from build123d import *

# Parameters (mm, degrees)
F1_DEPTH    = 25
F2_SIZE2    = 5
F2_SIZE     = 20
F3_SIZE2    = 5
F3_SIZE     = 20
F4_SIZE2    = 3
F4_SIZE     = 20
F5_SIZE2    = 10
F5_SIZE     = 20
F6_T1_DEPTH = 105.7467241961
F7_R        = 1.5
F13_DEPTH   = 80
F8_R        = 1.5
F14_DEPTH   = 30
F9_R        = 1.5
F15_DEPTH   = 40
F10_R       = 1.5
F16_DEPTH   = 30
F11_R       = 1.5
F17_DEPTH   = 80
F12_R       = 1.5
F18_DEPTH   = 55
F19_R       = 6
F25_DEPTH   = 12
F20_R       = 6
F26_DEPTH   = 12
F21_R       = 6
F27_DEPTH   = 12
F22_R       = 6
F28_DEPTH   = 12
F23_R       = 6
F29_DEPTH   = 12
F24_R       = 6
F30_DEPTH   = 12
F31_R       = 6
F34_D       = 4
F34_DEPTH   = 4
F34_TIP     = 1.2017212381


# Not quite as in the source:
# - a fillet or chamfer that OpenCascade refuses, or shapes differently, is made with other operations: its cross-section is extruded or revolved along the edge and cut away or added


with BuildPart() as f1:
    # F0 (on Top) → F1 (new body)
    with BuildSketch(Plane.XY):
        Polygon((15, 0), (4.6352549156, 14.2658477444), (-12.1352549156, 8.8167787844), (-12.1352549156, -8.8167787844), (4.6352549156, -14.2658477444), align=None)
    extrude(amount=F1_DEPTH)

    # F2
    f2_edges = [f1.edges().sort_by_distance(p)[0] for p in [
        (-3.75, -11.541313, 25),
    ]]
    f2_side = f1.faces().sort_by_distance((-3.75, -11.541313, 12.5))[0]
    chamfer(f2_edges, length=F2_SIZE, length2=F2_SIZE2, reference=f2_side)

    # F3
    f3_edges = [f1.edges().sort_by_distance(p)[0] for p in [
        (11.362712, -5.006297, 25),
    ]]
    f3_side = f1.faces().sort_by_distance((10.379872, -6.359061, 11.710138))[0]
    chamfer(f3_edges, length=F3_SIZE, length2=F3_SIZE2, reference=f3_side)

    # F4
    f4_edges = [f1.edges().sort_by_distance(p)[0] for p in [
        (8.272542, 9.259551, 25),
    ]]
    f4_side = f1.faces().sort_by_distance((9.255383, 7.906786, 11.710138))[0]
    chamfer(f4_edges, length=F4_SIZE, length2=F4_SIZE2, reference=f4_side)

    # F5
    f5_edges = [f1.edges().sort_by_distance(p)[0] for p in [
        (-5.25, 11.053934, 25),
    ]]
    f5_side = f1.faces().sort_by_distance((-4.319172, 11.356378, 12.050432))[0]
    chamfer(f5_edges, length=F5_SIZE, length2=F5_SIZE2, reference=f5_side)

    # F6: chamfer of 20 x 5 on 1 edges, made by hand

    # F6_s2 → F6_t1 (cut)
    with BuildSketch(Plane.XZ.offset(-50.2447065374)):
        Polygon((-12.1352549156, 5), (-7.1352549156, 25), (-12.1352549156, 25), align=None)
    extrude(amount=F6_T1_DEPTH, mode=Mode.SUBTRACT)

    # F7 (on face) → F13 (join)
    with BuildSketch(Plane(origin=(-12.5978869794, 0, 3.1494717449), x_dir=(0, -1, 0), z_dir=(-0.9701425001, 0, 0.242535625))):
        with Locations((0, 10.203753598)):
            Circle(F7_R)
    extrude(amount=F13_DEPTH)

    # F8 (on face) → F14 (join)
    with BuildSketch(Plane(origin=(-3.6180339887, 11.1351636441, 5.8541019662), x_dir=(-0.9610446388, -0.2446443083, -0.1286171243), z_dir=(-0.2763932023, 0.8506508084, 0.4472135955))):
        with Locations((-3.206722904, 8.4386551753)):
            Circle(F8_R)
    extrude(amount=F14_DEPTH)

    # F9 (on face) → F15 (join)
    with BuildSketch(Plane(origin=(10.1950026441, 7.4071029941, 1.8902574448), x_dir=(-0.5715412914, 0.8137020337, -0.1059695832), z_dir=(0.8000663158, 0.5812822037, 0.1483404529))):
        with Locations((-2.0448169671, 8.4398761392)):
            Circle(F9_R)
    extrude(amount=F15_DEPTH)

    # F10 (on face) → F16 (join)
    with BuildSketch(Plane(origin=(10.1919046596, -7.4048521765, 3.1494717449), x_dir=(0.5448158193, 0.8214813003, 0.168357347), z_dir=(0.7848617696, -0.5702354542, 0.242535625))):
        with Locations((2.4632040877, 6.1464309692)):
            Circle(F10_R)
    extrude(amount=F16_DEPTH)

    # F11 (on face) → F17 (join)
    with BuildSketch(Plane.XY.offset(25)):
        Circle(F11_R)
    extrude(amount=F17_DEPTH)

    # F12 (on face) → F18 (join)
    with BuildSketch(Plane(origin=(-3.8929611699, -11.9813025033, 3.1494717449), x_dir=(0.9540050547, -0.2899406279, 0.0762154044), z_dir=(-0.2997905195, -0.9226603465, 0.242535625))):
        with Locations((0, 17.0320216566)):
            Circle(F12_R)
    extrude(amount=F18_DEPTH)

    # F19 (on face) → F25 (join)
    with BuildSketch(Plane(origin=(-20.3814397429, -62.7276215607, 16.4889311219), x_dir=(0.9540050547, -0.2899406279, 0.0762154044), z_dir=(-0.2997905195, -0.9226603465, 0.242535625))):
        with Locations((0, 17.0320216566)):
            Circle(F19_R)
    extrude(amount=F25_DEPTH)

    # F20 (on face) → F26 (join)
    with BuildSketch(Plane(origin=(33.737757747, -24.5119158028, 10.4255404959), x_dir=(0.5448158193, 0.8214813003, 0.168357347), z_dir=(0.7848617696, -0.5702354542, 0.242535625))):
        with Locations((2.4632040877, 6.1464309692)):
            Circle(F20_R)
    extrude(amount=F26_DEPTH)

    # F21 (on face) → F27 (join)
    with BuildSketch(Plane(origin=(42.1976552771, 30.6583911409, 7.823875562), x_dir=(-0.5715412914, 0.8137020337, -0.1059695832), z_dir=(0.8000663158, 0.5812822037, 0.1483404529))):
        with Locations((-2.0448169671, 8.4398761392)):
            Circle(F21_R)
    extrude(amount=F27_DEPTH)

    # F22 (on face) → F28 (join)
    with BuildSketch(Plane(origin=(-11.9098300563, 36.6546878947, 19.2705098312), x_dir=(-0.9610446388, -0.2446443083, -0.1286171243), z_dir=(-0.2763932023, 0.8506508084, 0.4472135955))):
        with Locations((-3.206722904, 8.4386551753)):
            Circle(F22_R)
    extrude(amount=F28_DEPTH)

    # F23 (on face) → F29 (join)
    with BuildSketch(Plane(origin=(-90.209286991, 0, 22.5523217478), x_dir=(0, -1, 0), z_dir=(-0.9701425001, 0, 0.242535625))):
        with Locations((0, 10.203753598)):
            Circle(F23_R)
    extrude(amount=F29_DEPTH)

    # F24 (on face) → F30 (join)
    with BuildSketch(Plane.XY.offset(105)):
        Circle(F24_R)
    extrude(amount=F30_DEPTH)

    # F31
    f31_edges = [f1.edges().sort_by_distance(p)[0] for p in [
        (-99.376223, 6, 35.361844),
        (-6.378477, 45.188017, 33.290534),
        (-6, 0, 117),
        (54.85778, 31.087694, 18.754911),
        (-29.702956, -67.72987, 35.414485),
        (39.414513, -34.260153, 18.612961),
    ]]
    fillet(f31_edges, radius=F31_R)

    # F32: fillet of radius 5.9 on 6 edges, made by hand

    # F32_s1 → F32_t2 (revolve, cut)
    with BuildSketch(Plane(origin=(0, -3.9268533113, 7.4693188604), x_dir=(1, 0, 0), z_dir=(0, 0.4653411272, -0.8851314226))):
        with BuildLine():
            ThreePointArc((-10.2695931595, -41.8833034178), (-13.9610472636, -42.9942942584), (-16.1784394484, -46.1477536208))
            Line((-16.1784394484, -46.1477536208), (-14.594294034, -40.6395340077))
            Line((-14.594294034, -40.6395340077), (-10.2695931595, -41.8833034178))
        make_face()
    revolve(axis=Axis((-8.8280262013, 33.5123410902, 27.15226817), (-0.2763932023, 0.8506508084, 0.4472135955)), mode=Mode.SUBTRACT)

    # F32_s3 → F32_t4 (revolve, cut)
    with BuildSketch(Plane(origin=(-1.5386160993, 0, 8.2984438146), x_dir=(0, 1, 0), z_dir=(0.1823031611, 0, -0.9832423696))):
        with BuildLine():
            ThreePointArc((30.2150724668, 43.2335322221), (34.0656604389, 43.0488532565), (37.208345891, 45.2814889635))
            Line((37.208345891, 45.2814889635), (33.8767316186, 40.6177623056))
            Line((33.8767316186, 40.6177623056), (30.2150724668, 43.2335322221))
        make_face()
    revolve(axis=Axis((41.8277365078, 28.9945194162, 16.3390077783), (0.8000663158, 0.5812822037, 0.1483404529)), mode=Mode.SUBTRACT)

    # F32_s5 → F32_t6 (revolve, cut)
    with BuildSketch(Plane.XZ):
        with BuildLine():
            ThreePointArc((6, 110.7314919524), (4.7405818601, 107.0880046119), (1.5, 105))
            Line((1.5, 105), (6, 105))
            Line((6, 105), (6, 110.7314919524))
        make_face()
    revolve(axis=Axis((0, 0, 105), (0, 0, 1)), mode=Mode.SUBTRACT)

    # F32_s7 → F32_t8 (revolve, cut)
    with BuildSketch(Plane(origin=(-1.8146833973, 0, 5.8724388313), x_dir=(0, 1, 0), z_dir=(0.2952418088, 0, -0.9554225632))):
        with BuildLine():
            ThreePointArc((-21.2562177554, 37.5718299013), (-19.7847946135, 41.1349813138), (-20.8278518207, 44.8462029069))
            Line((-20.8278518207, 44.8462029069), (-17.559551904, 40.1378894452))
            Line((-17.559551904, 40.1378894452), (-21.2562177554, 37.5718299013))
        make_face()
    revolve(axis=Axis((33.2650669029, -22.4884397059, 16.7126778325), (0.7848617696, -0.5702354542, 0.242535625)), mode=Mode.SUBTRACT)

    # F32_s9 → F32_t10 (revolve, cut)
    with BuildSketch(Plane(origin=(0, 4.3300315839, 16.4724190146), x_dir=(1, 0, 0), z_dir=(0, -0.2542288679, -0.9671440858))):
        with BuildLine():
            ThreePointArc((-18.9504321609, 65.3082962809), (-16.4848646735, 68.2717589543), (-16.3756563646, 72.1252259123))
            Line((-16.3756563646, 72.1252259123), (-14.6574094147, 66.6573536187))
            Line((-14.6574094147, 66.6573536187), (-18.9504321609, 65.3082962809))
        make_face()
    revolve(axis=Axis((-20.3814397429, -58.3975899768, 32.9613501365), (-0.2997905195, -0.9226603465, 0.242535625)), mode=Mode.SUBTRACT)

    # F32_s11 → F32_t12 (revolve, cut)
    with BuildSketch(Plane(origin=(2.4747737566, 0, 9.8990950265), x_dir=(0, 1, 0), z_dir=(-0.242535625, 0, -0.9701425001))):
        with BuildLine():
            ThreePointArc((-1.5, -92.9856046689), (-4.7405818601, -95.0736092808), (-6, -98.7170966213))
            Line((-6, -98.7170966213), (-6, -92.9856046689))
            Line((-6, -92.9856046689), (-1.5, -92.9856046689))
        make_face()
    revolve(axis=Axis((-87.7345132344, 0, 32.4514167742), (-0.9701425001, 0, 0.242535625)), mode=Mode.SUBTRACT)

    # F34
    with Locations(Plane(origin=(0, 0, 0), x_dir=(1, 0, 0), z_dir=(0, 0, -1))):
        with Locations((0, 0)):
            Hole(F34_D / 2, depth=F34_DEPTH)
            with Locations((0, 0, -(F34_DEPTH + F34_TIP / 2))):  # 118° drill point
                Cone(0, F34_D / 2, F34_TIP, mode=Mode.SUBTRACT)


solid = f1.part
Design review of the part built by this model. Coordinates are the model's own, in mm. Coordinates: 2 decimals unless noted, no trailing zeros. Order: outer loops, then holes, each group sorted by start corner. A loop starts at its lowest first (then second) coordinate and runs counter-clockwise, first axis right, second up. Notation, with made-up numbers: M 71.5,85 L 94.5,85 A25 ccw 94.5,103 Z; hole C -30.75,23 d9. An arc over 180 degrees is marked long. Use a Markdown table: item, result.
(1) Add section A-A (z = 86.5). Give the boundary of the cut face in (x, y).
Worked answers:
| item | result |
|---|---|
| outline | C 0,0 d3 |
(2) Draft analysis for pull direction X (two halves, no side actions). For faces 1 (the cylindrical face through (-48.741, 0.325, 21.194)), 2 (the flat face through (9.89, 7.03, 2.47)), 3 (the flat face through (-3.867, -11.503, 2.465)), state which applies: released by +X, released by -X, zero draft, split by the parting line, or undercut.
Worked answers:
| item | result |
|---|---|
| face 1 | undercut |
| face 2 | released by +X |
| face 3 | released by -X |
(3) For P1, Ø12, axis at x = -2.5, y = 0, coming from the -Z side; P2, Ø6, axis at y = -32, z = 15.5, coming from the -X side; P3, Ø5.5, axis at y = 4, z = 3, coming from the -X side; P4, Ø6, axis at y = -21, z = 15.5, coming from the +X side, all flat-tipped, find the tip position at first contact; note any pin that passes through.
Worked answers:
| item | result |
|---|---|
| P1 | stops at z = 0 |
| P2 | stops at x = 33.1 |
| P3 | stops at x = -12.14 |
| P4 | stops at x = 43.39 |
(4) Wall thickness on probe 1 along Y at (x, z) = (0, 2); probe 2 along Y at (x, z) = (2, 106): over which ranges is each line inside the solid? List them lowest first.
Worked answers:
| item | result |
|---|---|
| probe 1 | y = -12.76 to -2, 2 to 12.76 |
| probe 2 | y = -3.02 to 3.02 |
